Source: three-view drawing plus pictorial views. Frame: mm from the lowest corner of the part. Coordinates: 2 decimals unless noted, no trailing zeros. Write each loop counter-clockwise with the first axis right and the second up, starting at its lowest first coordinate (ties: lowest second). Pieces come first, ordered by that corner, then holes. Notation, with made-up numbers: M 86,74 L 106,74 A15 cw 106,102 Z; hole C 64.25,42.5 d1. An arc over 180 degrees is marked long. Write item = value, one per line. Start each with the question number.
Item 1: Pull-direction query (Y, two-part tool) for the marked faces 1, 2 and 3; classes: +Y half, -Y half, draft (parallel to the pull), parting line (faces both ways), or undercut.
Item 2: Section C-C on z = 55.5. Output: boundary loops of the cut face in (x, y).
Item 3: Section A-A on y = 30. Output: boundary loops of the cut face in (x, z), plus the area to 3 significant figures.
Item 4: First-contact query: pin 1 Ø3 at (y, z) = (13, 43.5) entering from +X; pin 2 Ø2 at (x, z) = (45.5, 18) entering from +Y (3 decimals); pin 3 Ø12 at (x, z) = (53.5, 14) entering from -Y. Flat tips, straight axial feed; report the tip coordinate or a pass-through.
Item 5: Section D-D on y = 55.5. Output: boundary loops of the cut face in (x, z).
Item 6: Ray query, L1, parallel to X at y = 30, z = 12; L2, parallel to Y at x = 30, z = 32.5. Return the intervals inside material, ascending. Write a range as [from, to].
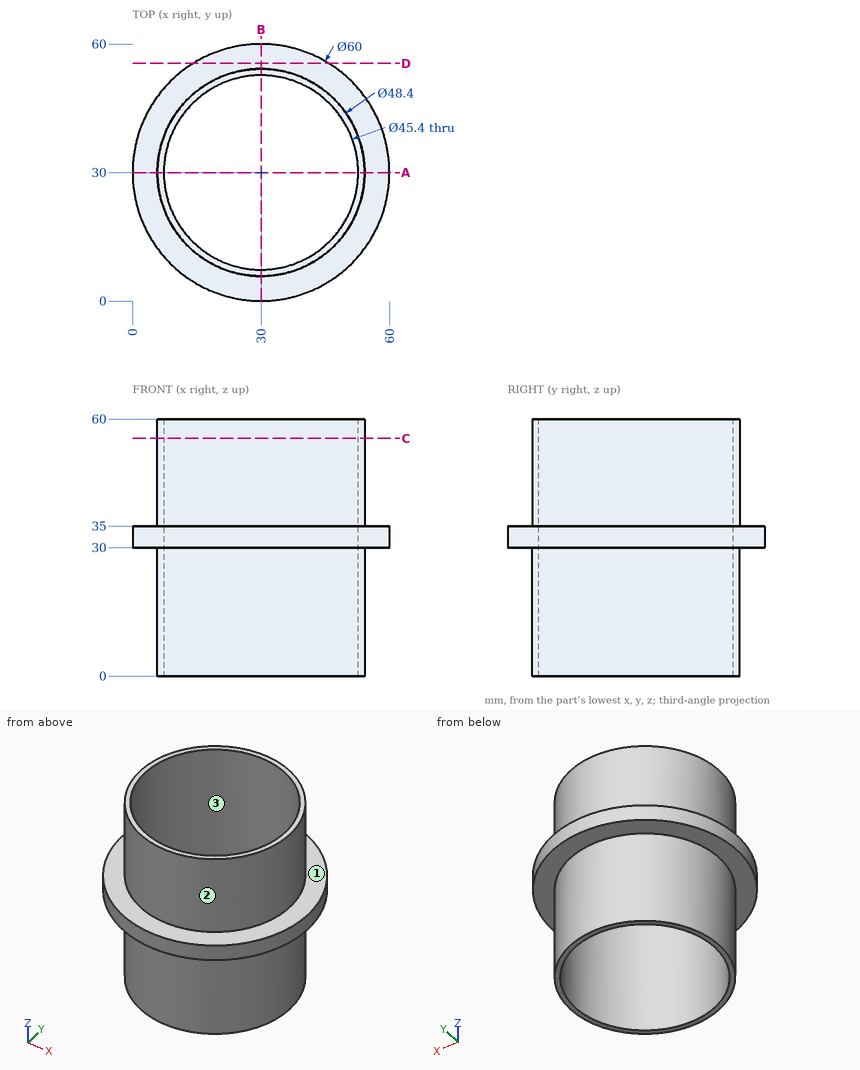
Responses:
q1.face_1 = draft
q1.face_2 = parting line
q1.face_3 = undercut
q2.outline = C 30,30 d48.4; hole C 30,30 d45.4
q3.outline = M 0,30 L 5.8,30 L 5.8,0 L 7.3,0 L 7.3,60 L 5.8,60 L 5.8,35 L 0,35 Z; M 52.7,0 L 54.2,0 L 54.2,30 L 60,30 L 60,35 L 54.2,35 L 54.2,60 L 52.7,60 Z
q3.area = 238 mm²
q4.pin_1 = 48.58
q4.pin_2 = 49.375
q4.pin_3 = 13.29
q5.outline = M 14.2,30 L 45.8,30 L 45.8,35 L 14.2,35 Z
q6.L1 = [5.8, 7.3], [52.7, 54.2]
q6.L2 = [0, 7.3], [52.7, 60]
